The listing builds one solid part. Answer for the finished solid, in the listing's coordinates (mm). A direction names the side the tool comes from. Give positions to 0.01 mm unless a question says otherwise; leave off trailing zeros. Write each loop counter-clockwise with the first axis right and the second up, starting at its lowest first coordinate (ties: lowest second). Pieces come first, ordered by that corner, then holes. Notation, with made-up numbers: M 0.5,-31.5 L 55.5,-31.5 A28 ccw 55.5,-6.5 Z; hole C -15,-33 d4. An arc over 180 degrees is marked long. Return JSON: item names as keys, results as strings.
from build123d import *

# Parameters (mm, degrees)
PLACA_DELANTERA_START               = 203
PLACA_DELANTERA_DEPTH               = 3
AGUJERO_PLACA_DELANTERA_1_PROFILE_R = 2
AGUJERO_PLACA_DELANTERA_2_PROFILE_R = 2
AGUJERO_PLACA_DELANTERA_3_PROFILE_R = 2
AGUJERO_PLACA_DELANTERA_4_PROFILE_R = 2
PLACA_TRASERA_START                 = 139
PLACA_TRASERA_DEPTH                 = 3
AGUJERO_PLACA_TRASERA_1_PROFILE_R   = 2
AGUJERO_PLACA_TRASERA_2_PROFILE_R   = 2
AGUJERO_PLACA_TRASERA_3_PROFILE_R   = 2
AGUJERO_PLACA_TRASERA_4_PROFILE_R   = 2
MARCO_INTERIOR_START                = 86
SK_MARCO_INTERIOR_W                 = 64
SK_MARCO_INTERIOR_H                 = 26
SK_MARCO_INTERIOR_R                 = 11
MARCO_INTERIOR_DEPTH                = 3
MARCO_EXTERIOR_START                = 143
SK_MARCO_EXTERIOR_W                 = 64
SK_MARCO_EXTERIOR_H                 = 26
SK_MARCO_EXTERIOR_R                 = 11
MARCO_EXTERIOR_DEPTH                = 3
CROQUIS17_W                         = 25.795648089
CROQUIS17_H                         = 11.561302328
CORTAR_EXTRUIR1_DEPTH               = 10


with BuildPart() as part:
    # Sk_Eje_cuerpo → Eje_cuerpo (revolve)
    with BuildSketch(Plane(origin=(0, 0, 0), x_dir=(1, 0, 0), z_dir=(0, 1, 0)), mode=Mode.PRIVATE) as eje_cuerpo_sk:
        Polygon((183.5, -84), (186, -84), (186, -92), (182.5, -92), (182.5, -138), (186, -138), (186, -146), (185.3, -149), (183.3, -152), (180, -154.5), (176.5, -155.7), (172.5, -156), (172.5, -147), (183.5, -147), (183.5, -138.5), (178.8, -138.5), (178.8, -91.5), (183.5, -91.5), align=None)
    revolve(eje_cuerpo_sk.sketch.rotate(Axis((172.5, 0, 62.1), (0, 0, 1)), 180), axis=Axis((172.5, 0, 62.1), (0, 0, 1)))



with BuildPart() as body_2:
    # Sk_Placa_delantera → Placa_delantera (new body)
    with BuildSketch(Plane(origin=(0, 0, 0), x_dir=(0, 0, -1), z_dir=(1, 0, 0)).offset(PLACA_DELANTERA_START)):
        Polygon((-86, -12), (-112, -12), (-116, -22), (-120, -12), (-146, -12), (-146, 10), (-144.125, 14), (-142.25, 10), (-140.375, 14), (-138.5, 10), (-136.625, 14), (-134.75, 10), (-132.875, 14), (-131, 10), (-129.125, 14), (-127.25, 10), (-125.375, 14), (-123.5, 10), (-121.625, 14), (-119.75, 10), (-117.875, 14), (-116, 10), (-114.125, 14), (-112.25, 10), (-110.375, 14), (-108.5, 10), (-106.625, 14), (-104.75, 10), (-102.875, 14), (-101, 10), (-99.125, 14), (-97.25, 10), (-95.375, 14), (-93.5, 10), (-91.625, 14), (-89.75, 10), (-87.875, 14), (-86, 10), align=None)
    extrude(amount=PLACA_DELANTERA_DEPTH)

    # Agujero_Placa_delantera_1: sweep along a curve in space
    with BuildLine() as agujero_placa_delantera_1_path:
        Line((201.5, -6, 91), (207.5, -6, 91))
    # Agujero_Placa_delantera_1 profile (on start of the path) → Agujero_Placa_delantera_1 (sweep, cut)
    with BuildSketch(Plane(origin=(201.5, -6, 91), x_dir=(0, 0, 1), z_dir=(1, 0, 0))):
        Circle(AGUJERO_PLACA_DELANTERA_1_PROFILE_R)
    sweep(path=agujero_placa_delantera_1_path.line, mode=Mode.SUBTRACT)

    # Agujero_Placa_delantera_2: sweep along a curve in space
    with BuildLine() as agujero_placa_delantera_2_path:
        Line((201.5, 2, 91), (207.5, 2, 91))
    # Agujero_Placa_delantera_2 profile (on start of the path) → Agujero_Placa_delantera_2 (sweep, cut)
    with BuildSketch(Plane(origin=(201.5, 2, 91), x_dir=(0, 0, 1), z_dir=(1, 0, 0))):
        Circle(AGUJERO_PLACA_DELANTERA_2_PROFILE_R)
    sweep(path=agujero_placa_delantera_2_path.line, mode=Mode.SUBTRACT)

    # Agujero_Placa_delantera_3: sweep along a curve in space
    with BuildLine() as agujero_placa_delantera_3_path:
        Line((201.5, -6, 141), (207.5, -6, 141))
    # Agujero_Placa_delantera_3 profile (on start of the path) → Agujero_Placa_delantera_3 (sweep, cut)
    with BuildSketch(Plane(origin=(201.5, -6, 141), x_dir=(0, 0, 1), z_dir=(1, 0, 0))):
        Circle(AGUJERO_PLACA_DELANTERA_3_PROFILE_R)
    sweep(path=agujero_placa_delantera_3_path.line, mode=Mode.SUBTRACT)

    # Agujero_Placa_delantera_4: sweep along a curve in space
    with BuildLine() as agujero_placa_delantera_4_path:
        Line((201.5, 2, 141), (207.5, 2, 141))
    # Agujero_Placa_delantera_4 profile (on start of the path) → Agujero_Placa_delantera_4 (sweep, cut)
    with BuildSketch(Plane(origin=(201.5, 2, 141), x_dir=(0, 0, 1), z_dir=(1, 0, 0))):
        Circle(AGUJERO_PLACA_DELANTERA_4_PROFILE_R)
    sweep(path=agujero_placa_delantera_4_path.line, mode=Mode.SUBTRACT)


with BuildPart() as body_3:
    # Sk_Placa_trasera → Placa_trasera (new body)
    with BuildSketch(Plane(origin=(0, 0, 0), x_dir=(0, 0, -1), z_dir=(1, 0, 0)).offset(PLACA_TRASERA_START)):
        Polygon((-86, -12), (-146, -12), (-146, 10), (-144.125, 14), (-142.25, 10), (-140.375, 14), (-138.5, 10), (-136.625, 14), (-134.75, 10), (-132.875, 14), (-131, 10), (-129.125, 14), (-127.25, 10), (-125.375, 14), (-123.5, 10), (-121.625, 14), (-119.75, 10), (-117.875, 14), (-116, 10), (-114.125, 14), (-112.25, 10), (-110.375, 14), (-108.5, 10), (-106.625, 14), (-104.75, 10), (-102.875, 14), (-101, 10), (-99.125, 14), (-97.25, 10), (-95.375, 14), (-93.5, 10), (-91.625, 14), (-89.75, 10), (-87.875, 14), (-86, 10), align=None)
    extrude(amount=PLACA_TRASERA_DEPTH)

    # Agujero_Placa_trasera_1: sweep along a curve in space
    with BuildLine() as agujero_placa_trasera_1_path:
        Line((137.5, -6, 91), (143.5, -6, 91))
    # Agujero_Placa_trasera_1 profile (on start of the path) → Agujero_Placa_trasera_1 (sweep, cut)
    with BuildSketch(Plane(origin=(137.5, -6, 91), x_dir=(0, 0, 1), z_dir=(1, 0, 0))):
        Circle(AGUJERO_PLACA_TRASERA_1_PROFILE_R)
    sweep(path=agujero_placa_trasera_1_path.line, mode=Mode.SUBTRACT)

    # Agujero_Placa_trasera_2: sweep along a curve in space
    with BuildLine() as agujero_placa_trasera_2_path:
        Line((137.5, 2, 91), (143.5, 2, 91))
    # Agujero_Placa_trasera_2 profile (on start of the path) → Agujero_Placa_trasera_2 (sweep, cut)
    with BuildSketch(Plane(origin=(137.5, 2, 91), x_dir=(0, 0, 1), z_dir=(1, 0, 0))):
        Circle(AGUJERO_PLACA_TRASERA_2_PROFILE_R)
    sweep(path=agujero_placa_trasera_2_path.line, mode=Mode.SUBTRACT)

    # Agujero_Placa_trasera_3: sweep along a curve in space
    with BuildLine() as agujero_placa_trasera_3_path:
        Line((137.5, -6, 141), (143.5, -6, 141))
    # Agujero_Placa_trasera_3 profile (on start of the path) → Agujero_Placa_trasera_3 (sweep, cut)
    with BuildSketch(Plane(origin=(137.5, -6, 141), x_dir=(0, 0, 1), z_dir=(1, 0, 0))):
        Circle(AGUJERO_PLACA_TRASERA_3_PROFILE_R)
    sweep(path=agujero_placa_trasera_3_path.line, mode=Mode.SUBTRACT)

    # Agujero_Placa_trasera_4: sweep along a curve in space
    with BuildLine() as agujero_placa_trasera_4_path:
        Line((137.5, 2, 141), (143.5, 2, 141))
    # Agujero_Placa_trasera_4 profile (on start of the path) → Agujero_Placa_trasera_4 (sweep, cut)
    with BuildSketch(Plane(origin=(137.5, 2, 141), x_dir=(0, 0, 1), z_dir=(1, 0, 0))):
        Circle(AGUJERO_PLACA_TRASERA_4_PROFILE_R)
    sweep(path=agujero_placa_trasera_4_path.line, mode=Mode.SUBTRACT)


with BuildPart() as part_1:
    add(part.part)

    add(body_2.part)  # Marco_interior merges body 2

    add(body_3.part)  # Marco_interior merges body 3
    # Sk_Marco_interior → Marco_interior (add)
    with BuildSketch(Plane.XY.offset(MARCO_INTERIOR_START)):
        with Locations((172.5, 0)):
            Rectangle(SK_MARCO_INTERIOR_W, SK_MARCO_INTERIOR_H)
        with Locations(Location((172.5, 0, 0), (0, 0, 180))):
            Circle(SK_MARCO_INTERIOR_R, mode=Mode.SUBTRACT)
    extrude(amount=MARCO_INTERIOR_DEPTH)

    # Sk_Marco_exterior → Marco_exterior (add)
    with BuildSketch(Plane.XY.offset(MARCO_EXTERIOR_START)):
        with Locations((172.5, 0)):
            Rectangle(SK_MARCO_EXTERIOR_W, SK_MARCO_EXTERIOR_H)
        with Locations(Location((172.5, 0, 0), (0, 0, 180))):
            Circle(SK_MARCO_EXTERIOR_R, mode=Mode.SUBTRACT)
    extrude(amount=MARCO_EXTERIOR_DEPTH)

    # Croquis17 → Cortar-Extruir1 (cut)
    with BuildSketch(Plane(origin=(206, 0, 0), x_dir=(0, 0, -1), z_dir=(1, 0, 0))):
        with Locations((-104.897824044, -1.951399644)):
            Rectangle(CROQUIS17_W, CROQUIS17_H)
    cortar_extruir1 = extrude(amount=-CORTAR_EXTRUIR1_DEPTH, mode=Mode.SUBTRACT)

    # Simetr_a1: Cortar-Extruir1 across plane
    add(cortar_extruir1.mirror(Plane(origin=(172, 0, 0), x_dir=(0, 0, 1), z_dir=(1, 0, 0))), mode=Mode.SUBTRACT)


solid = part_1.part
Item 1: A cutting plane is placed at A-A, the plane x = 146. Write down the section's boundary in (y, z), plus the area to 3 significant figures.
Geometry results:
{"outline": "M -13,86 L 13,86 L 13,89 L -13,89 Z; M -13,143 L 13,143 L 13,146 L -13,146 Z", "area": "156 mm2"}
Item 2: Determine the mould class of faces 1 (the cylindrical face through (163.263, 3.83, 115.322)), 2 (the flat face through (150, 0, 146)) for opening direction X: +X half, -X half, draft (parallel to the pull), parting line (faces both ways), or undercut.
Geometry results:
{"face 1": "undercut", "face 2": "draft"}
Item 3: A cutting plane is placed at C-C, the plane y = 8.5. Count the separate pieces of the cut face and the enclosed holes in it, plus the area to 3 significant figures.
Geometry results:
{"separate pieces": "1", "enclosed holes": "3", "area": "1,320 mm2"}
Item 4: A cutting plane is placed at B-B, the plane z = 94.5. Write down the section's boundary in (x, y), plus the area to 3 significant figures.
Geometry results:
{"outline": "M 139,-12 L 142,-12 L 142,-7.73 L 139,-7.73 Z; M 139,3.83 L 142,3.83 L 142,12.13 L 139,12.13 Z; C 172.5,0 d20; M 203,-12 L 206,-12 L 206,-7.73 L 203,-7.73 Z; M 203,3.83 L 206,3.83 L 206,12.13 L 203,12.13 Z; hole C 172.5,0 d12.6", "area": "265 mm2"}
Item 5: Given pin 1 Ø0.9 at (x, y) = (140, -1.5) entering from +Z; pin 2 Ø11 at (x, y) = (167, 5.5) entering from -Z; pin 3 Ø1.5 at (x, y) = (163.5, -1.5) entering from +Z; pin 4 Ø1.5 at (x, z) = (155.5, 87.5) entering from -Y, each flat-ended and moving along its own axis, determine where each tip first touches the part or whether it passes through.
Geometry results:
{"pin 1": "stops at z = 146", "pin 2": "stops at z = 84", "pin 3": "stops at z = 153.84", "pin 4": "stops at y = -13"}
Item 6: Which of the six approach directions +Z, -Z, +X, -X, +Y, -Y give full straight-line access (tool end or side, diameter ignored) to faces 3 (the flat face through (140, -7.732, 105)), 4 (the flat face through (183, 0, 92)), 5 (the flat face through (203, 0, 122)), 6 (the cylindrical face through (178.794, -0.277, 114.671))?
Geometry results:
{"face 3": "-X", "face 4": "none", "face 5": "+Y, -Y", "face 6": "-Z"}
Item 7: Find the intervals of material crossed by line 1 (Z direction, x = 140, y = 2); line 2 (X direction, y = -11.5, z = 101); line 3 (Z direction, x = 190, y = -10.5), in increasing order.
Geometry results:
{"line 1": "z = 86 to 89, 117.8 to 139, 143 to 146", "line 2": "x = 139 to 142, 203 to 206", "line 3": "z = 86 to 89, 143 to 146"}
